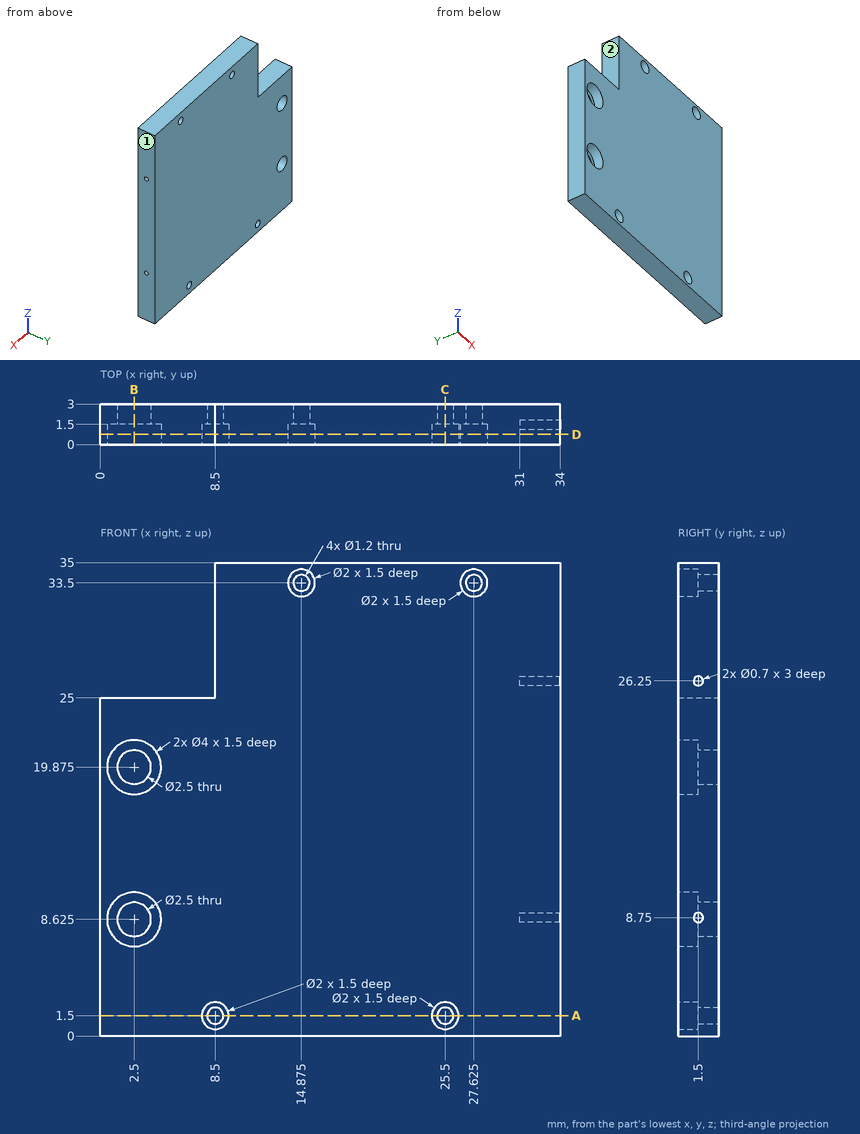
Source: three-view drawing plus pictorial views. Frame: mm from the lowest corner of the part. A direction names the side the tool comes from. Round coordinates to 2 decimals unless told otherwise and drop trailing zeros. Loops run counter-clockwise (first coordinate to the right, second up) from the corner with the lowest first, then second, coordinate; pieces in that order, holes last.
Item 1: Reachability of the marked faces 1 and 2 from +Z, -Z, +X, -X, +Y, -Y: full face, straight path, thin tool, end or side. Return the list, or none.
Checked values:
face 1: +Z, -Z, +X, +Y, -Y
face 2: +Z, -X, +Y, -Y
Item 2: Section C-C, the plane x = 25.5. Output: boundary loops of the cut face in (y, z).
Checked values:
outline: (0, 0) - (3, 0) - (3, 0.9) - (1.5, 0.9) - (1.5, 0.5) - (0, 0.5) - close; (0, 2.5) - (1.5, 2.5) - (1.5, 2.1) - (3, 2.1) - (3, 35) - (0, 35) - close
Item 3: Section D-D, the plane y = 0.75. Output: boundary loops of the cut face in (x, z) (3 decimals), plus the area to 3 significant figures.
Checked values:
outline: (0, 0) - (34, 0) - (34, 35) - (8.5, 35) - (8.5, 25) - (0, 25) - close; hole circle Ø4 at (2.5, 8.625); hole circle Ø4 at (2.5, 19.875); hole circle Ø2 at (8.5, 1.5); hole circle Ø2 at (14.875, 33.5); hole circle Ø2 at (25.5, 1.5); hole circle Ø2 at (27.625, 33.5)
area: 1,070 mm2
Item 4: Line query: L1, parallel to X at y = 2.25, z = 1.5; L2, parallel to X at y = 2.5, z = 33.5 (3 decimals); L3, parallel to Z at x = 6.5, y = 2.7. Output: solid intervals per line, ascending.
Checked values:
L1: x = 0 to 7.9, 9.1 to 24.9, 26.1 to 34
L2: x = 8.5 to 14.275, 15.475 to 27.025, 28.225 to 34
L3: z = 0 to 25
Item 5: Section B-B, the plane x = 2.5. Output: boundary loops of the cut face in (y, z) (3 decimals).
Checked values:
outline: (0, 0) - (3, 0) - (3, 7.375) - (1.5, 7.375) - (1.5, 6.625) - (0, 6.625) - close; (0, 10.625) - (1.5, 10.625) - (1.5, 9.875) - (3, 9.875) - (3, 18.625) - (1.5, 18.625) - (1.5, 17.875) - (0, 17.875) - close; (0, 21.875) - (1.5, 21.875) - (1.5, 21.125) - (3, 21.125) - (3, 25) - (0, 25) - close
Item 6: Contact query for flat-ended pins moving along their axis: P1, Ø1, axis at x = 25.5, z = 1.5, coming from the +Y side; P2, Ø0.6, axis at x = 27.5, z = 33, coming from the -Y side; P3, Ø0.9, axis at y = 2, z = 29.5, coming from the -X side. Output: stop coordinate, or through.
Checked values:
P1: passes through
P2: stops at y = 1.5
P3: stops at x = 8.5
Item 7: Section A-A, the plane z = 1.5. Output: boundary loops of the cut face in (x, y), plus the area to 3 significant figures.
Checked values:
outline: (0, 0) - (7.5, 0) - (7.5, 1.5) - (7.9, 1.5) - (7.9, 3) - (0, 3) - close; (9.1, 1.5) - (9.5, 1.5) - (9.5, 0) - (24.5, 0) - (24.5, 1.5) - (24.9, 1.5) - (24.9, 3) - (9.1, 3) - close; (26.1, 1.5) - (26.5, 1.5) - (26.5, 0) - (34, 0) - (34, 3) - (26.1, 3) - close
area: 92.4 mm2
